from build123d import *
from build123d import SkipClean  # not in build123d's __all__

# Parameters (mm, degrees)
F0_R             = 19.5
F0_R_2           = 14.5
F1_DEPTH         = 40
F2_R             = 17
F3_DEPTH         = 30
F5_R             = 19.5
F6_COPIES_COUNT  = 3
F8_END_RADIUS    = 17
F7_R             = 14.5
F8_REACH         = 132.9006886826
F8_COPIES_COUNT  = 3
F8_COPIES_ANGLE  = 239.9998
F9_R             = 17
F10_DEPTH        = 30
F10_COPIES_COUNT = 3


# Not quite as in the source:
# - a pattern or mirror of a feature is missing from the dataset's text; its kind, count and spacing are read off the source's solid


with BuildPart() as f1:
    # F0 (on Top) → F1 (new body)
    with BuildSketch(Plane.XY):
        Circle(F0_R)
        Circle(F0_R_2, mode=Mode.SUBTRACT)
    extrude(amount=F1_DEPTH)

    # F2 (on face) → F3 (cut)
    with BuildSketch(Plane.XY.offset(40)):
        Circle(F2_R)
    extrude(amount=-F3_DEPTH, mode=Mode.SUBTRACT)

    # F5 (on offset) → F6 (join, up to the next surface of F1)
    with BuildSketch(Plane.XZ.offset(50)):
        with Locations((0, 19.5)):
            Circle(F5_R)
    with SkipClean():  # cleaning this boolean's faces spoils the solid; the shape is the same uncleaned
        f6 = extrude(until=Until.NEXT, dir=(0, 1, 0))

    # F6_copies: F6 ×3 about axis
    f6_copies_axis = Axis((0, 0, 0), (0, 0, 1))
    for i in range(1, F6_COPIES_COUNT):
        add(f6.rotate(f6_copies_axis, i * 360 / F6_COPIES_COUNT), clean=False)

    f8_end = (Plane.XY.offset(25) * Cylinder(F8_END_RADIUS, 557.6990366969, mode=Mode.PRIVATE)).faces().sort_by_distance((-17, 0, 25))[0]
    # F7 (on offset) → F8 (cut, up to the whole of a round face its end follows)
    with BuildSketch(Plane.XZ.offset(50)):
        with Locations((0, 19.5)):
            Circle(F7_R)
    f8_long = extrude(amount=-F8_REACH, mode=Mode.PRIVATE)
    f8 = split(f8_long, bisect_by=f8_end, keep=Keep.ALL, mode=Mode.PRIVATE).solids().sort_by_distance((0, -50, 19.5))[0]
    add(f8, mode=Mode.SUBTRACT)

    # F8_copies: F8 ×3 about axis
    f8_copies_axis = Axis((0, 0, 0), (0, 0, 1))
    for i in range(1, F8_COPIES_COUNT):
        add(f8.rotate(f8_copies_axis, i * F8_COPIES_ANGLE / (F8_COPIES_COUNT - 1)), clean=False, mode=Mode.SUBTRACT)

    # F9 (on offset) → F10 (cut)
    with BuildSketch(Plane.XZ.offset(50)):
        with Locations((0, 19.5)):
            Circle(F9_R)
    f10 = extrude(amount=-F10_DEPTH, mode=Mode.SUBTRACT)

    # F10_copies: F10 ×3 about axis
    f10_copies_axis = Axis((0, 0, 0), (0, 0, 1))
    for i in range(1, F10_COPIES_COUNT):
        add(f10.rotate(f10_copies_axis, i * 360 / F10_COPIES_COUNT), clean=False, mode=Mode.SUBTRACT)


solid = f1.part
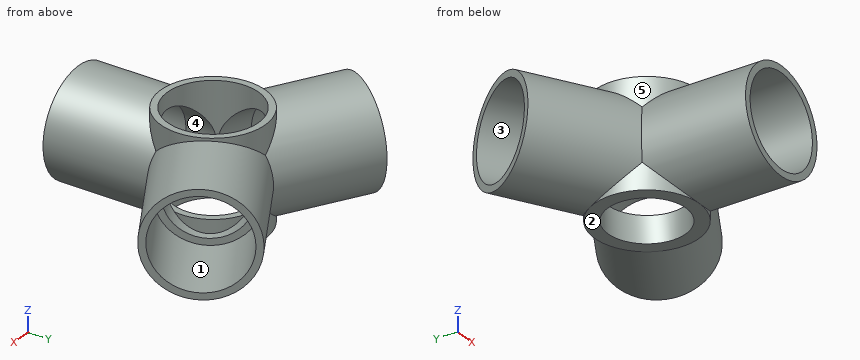
Model file for the job. Use its own axes, mm. Face numbers are marked on the shaded views. A direction names the side the tool comes from. Give positions to 0.01 mm unless a question says otherwise; leave off trailing zeros. Order: outer loops, then holes, each group sorted by start corner. A loop starts at its lowest first (then second) coordinate and runs counter-clockwise, first axis right, second up. Notation, with made-up numbers: (69.5, -28.75) - (108.5, -28.75) arc R23 cw to (108.5, -11.75) - close; hole circle Ø4 at (-6, -9.5). An arc over 180 degrees is marked (long way). Return JSON: item names as keys, results as strings.
1) Cut at C-C, the plane y = -31.5. Give the cut face in (x, z), plus the area to 3 significant figures.
Geometry says:
{"outline": "circle Ø39 at (0, 19.5); hole circle Ø34 at (0, 19.5)", "area": "287 mm²"}
2) 3-axis set-ups, long thin cutter, end or side, ignore diameter. For the marked faces 3, 4 and 5: which of +Z, -Z, +X, -X, +Y, -Y reach the whole face in a straight line?
Geometry says:
{"face 3": "none", "face 4": "-Y", "face 5": "+Z"}
3) Flat gauge pins, fed straight in: P1, Ø12, axis at y = -26, z = 4, coming from the +X side; P2, Ø3, axis at x = -21, z = 8, coming from the -Y side; P3, Ø10, axis at x = 11.5, z = 11, coming from the +Y side; P4, Ø17.5, axis at x = 0, y = 0, coming from the +Z side. Where does each tip first touch, or does it go through?
Geometry says:
{"P1": "x = 17.03", "P2": "y = -7.52", "P3": "y = 30.57", "P4": "through"}
4) Pull direction Y, two halves, no side cores. Call the marked faces 1 and 2: pulls with the +Y half, pulls with the -Y half, needs draft (parallel to the pull), parting line crosses it, or undercut.
Geometry says:
{"face 1": "undercut", "face 2": "needs draft"}
5) Cut at A-A, the plane z = 25.5. Count the separate pieces of the cut face and the enclosed holes in it, plus the area to 3 significant figures.
Geometry says:
{"separate pieces": "3", "enclosed holes": "0", "area": "810 mm²"}
6) Probe line 1 (X direction, y = -12.25, z = 19.5); line 2 (Y direction, x = 0, z = 5.5); line 3 (Z direction, x = 30, y = 25). List the from-to ranges inside material, lowest first. Write a range as from..to.
Geometry says:
{"line 1": "-19.5..-14.5, 14.5..19.5", "line 2": "-17..-14.5, 14.5..19.5", "line 3": "1.17..3.85, 35.15..37.83"}
